Could you check a few things on this model? Use its own coordinates, in mm. Face numbers are marked on the shaded views. Coordinates: 2 decimals unless noted, no trailing zeros. Write each loop counter-clockwise with the first axis right and the second up, starting at its lowest first coordinate (ties: lowest second). Pieces come first, ordered by that corner, then holes.
```python
from build123d import *
from build123d.topology import SkipClean

# Parameters (mm, degrees)
DODANIE_WYCI_GNI_CIE1_DEPTH = 8
SZKIC2_R                    = 2
WYTNIJ_WYCI_GNI_CIE1_DEPTH  = 8
ZAOKR_GLENIE1_R             = 0.5


with BuildPart() as part:
    # Szkic1 → Dodanie-wyciągnięcie1 (new body)
    with BuildSketch(Plane.XY):
        with BuildLine():
            Line((0, 0.876524617), (0, -0.123475383))
            ThreePointArc((0, -0.123475383), (2.035134096, -0.3133769), (4, -0.876524617))
            Line((4, -0.876524617), (4, 0.876524617))
            Line((4, 0.876524617), (0, 0.876524617))
        make_face()
        with BuildLine():
            ThreePointArc((-4, -0.876524617), (-2.035134096, -0.3133769), (0, -0.123475383))
            Line((0, -0.123475383), (0, 0.876524617))
            Line((0, 0.876524617), (-4, 0.876524617))
            Line((-4, 0.876524617), (-4, -0.876524617))
        make_face()
    extrude(amount=DODANIE_WYCI_GNI_CIE1_DEPTH)

    # Szkic2 → Wytnij-wyciągnięcie1 (cut)
    with SkipClean():  # the faces are left unmerged after this step: merging them gives an invalid solid
        with BuildSketch(Plane(origin=(0, 0.876524617, 0), x_dir=(1, 0, 0), z_dir=(0, 1, 0))):
            with Locations(Location((0, -4, 0), (0, 0, 270))):
                Circle(SZKIC2_R)
        extrude(amount=-WYTNIJ_WYCI_GNI_CIE1_DEPTH, mode=Mode.SUBTRACT)

    # Zaokrąglenie1
    zaokr_glenie1_edges = [part.edges().sort_by_distance(p)[0] for p in [
        (4, 0, 8),
        (-4, 0, 8),
        (-4, 0, 0),
        (4, 0, 0),
    ]]
    fillet(zaokr_glenie1_edges, radius=ZAOKR_GLENIE1_R)


solid = part.part
```
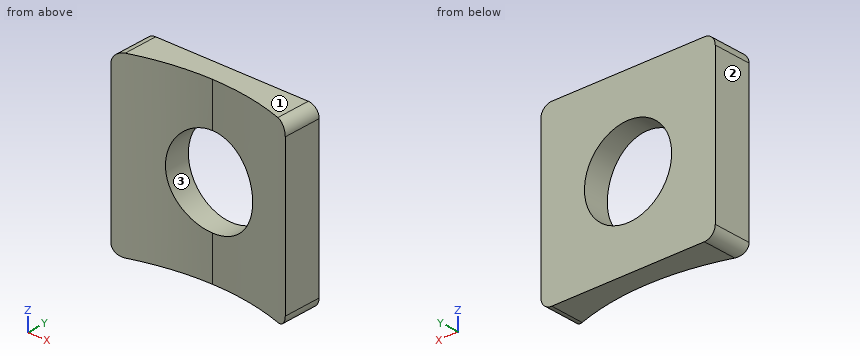
1. I want a section at D-D on z = 7. Please give me the cut outline in (x, y).
Verdict:
outline: (-4, -0.88) arc R11 cw to (4, -0.88) - (4, 0.88) - (-4, 0.88) - close
2. I want a section at C-C on x = -1.5. Please give me the cut outline in (y, z), plus the area to 3 significant figures.
Verdict:
outline: (-0.23, 0) - (0.88, 0) - (0.88, 2.68) - (-0.23, 2.68) - close; (-0.23, 5.32) - (0.88, 5.32) - (0.88, 8) - (-0.23, 8) - close
area: 5.90 mm2
3. I want a section at B-B on z = 4. Please give me the cut outline in (x, y).
Verdict:
outline: (-4, -0.88) arc R11 cw to (-2, -0.31) - (-2, 0.88) - (-4, 0.88) - close; (2, -0.31) arc R11 cw to (4, -0.88) - (4, 0.88) - (2, 0.88) - close
4. I want a section at A-A on y = 0.4. Please give me the cut outline in (x, z).
Verdict:
outline: (-4, 0.5) arc R0.5 ccw to (-3.5, 0) - (3.5, 0) arc R0.5 ccw to (4, 0.5) - (4, 7.5) arc R0.5 ccw to (3.5, 8) - (-3.5, 8) arc R0.5 ccw to (-4, 7.5) - close; hole circle Ø4 at (0, 4)
5. Please list where these lines run through material, in increasing order: line 1 along X through (y, z) = (0.6, 4); line 2 along Y through (x, z) = (3.5, 4); line 3 along Y through (x, z) = (-2, 1).
Verdict:
line 1: x = -4 to -2, 2 to 4
line 2: y = -0.7 to 0.88
line 3: y = -0.31 to 0.88
6. If we mould it in two halves opening along Z, with no side actions, what happens to the marked faces 1, 2 and 3? For each: pulls with the +Z half, pulls with the -Z half, needs draft (parallel to the pull), parting line crosses it, or undercut.
Verdict:
face 1: pulls with the +Z half
face 2: needs draft
face 3: undercut
